Input: part model. Units: mm. Frame: model coordinates. A direction names the side the tool comes from. Round coordinates to 2 decimals unless told otherwise and drop trailing zeros. Write each loop counter-clockwise with the first axis right and the second up, starting at its lowest first coordinate (ties: lowest second). Pieces come first, ordered by that corner, then holes. Notation, with made-up numbers: (58, 24.25) - (116, 24.25) arc R14 ccw to (116, 28.25) - close; hole circle Ø5 at (-9, 30.5). An arc over 180 degrees is marked (long way). One line per item, written item: value. Start each with the question number.
```python
from build123d import *

# Parameters (mm, degrees)
BOSS_EXTRUDE1_DEPTH     = 6.35
F_3_8_CLEARANCE_HOLE1_D = 10.0838
BODY_MOVE_COPY2_ANGLE   = 90
F_1_4_CLEARANCE_HOLE1_D = 6.7564
SKETCH6_W               = 11.2395
SKETCH6_H               = 11.2395
CUT_EXTRUDE1_DEPTH      = 6.8326
F_3_8_CLEARANCE_HOLE3_D = 10.0838
FILLET1_R               = 3.175
F_3_8_CLEARANCE_HOLE2_D = 13.97


with BuildPart() as part:
    # Sketch2 → Boss-Extrude1 (new, symmetric)
    with BuildSketch(Plane.XY):
        Polygon((-25.4, -25.4), (25.4, -25.4), (25.4, 50.8), (12.7, 76.2), (-12.7, 76.2), (-25.4, 50.8), align=None)
    extrude(amount=BOSS_EXTRUDE1_DEPTH, both=True)

    # 3/8 Clearance Hole1 (through all)
    with Locations(Plane.XY.offset(6.35)):
        with Locations((0, 0), (0, 57.15)):
            Hole(F_3_8_CLEARANCE_HOLE1_D / 2)


with BuildPart() as body_2:
    # uxcell-FR6ZZ: read off the stored shape, not the designer's step
    # uxcell-FR6ZZ outline → uxcell-FR6ZZ (revolve)
    with BuildSketch(Plane(origin=(-48.38860798, 0, 0), x_dir=(1, 0, 0), z_dir=(0, 0, 1))):
        Polygon((12.430125, 12.468326067), (4.7625, 12.468326067), (4.7625, 4.054576067), (11.2395, 4.054576067), (11.2395, 9.213951067), (11.636375, 9.610826067), (12.430125, 9.610826067), align=None)
    revolve(axis=Axis((-48.38860798, 0, 0), (0, 1, 0)))


with BuildPart() as body_2_1:
    # Body-Move/Copy2: read off the stored shape, not the designer's step
    # Body-Move/Copy2: moved
    add(body_2.part.moved(Location((48.388608, -6.1183261, 0))).rotate(Axis((0, 0, 0), (1, 0, 0)), BODY_MOVE_COPY2_ANGLE))


with BuildPart() as part_1:
    add(part.part)

    # Combine1: cut body 2
    add(body_2_1.part, mode=Mode.SUBTRACT)

    # 1/4 Clearance Hole1 (through all)
    with Locations(Plane.XY.offset(6.35)):
        with Locations((-15.875, 15.875), (15.875, 15.875), (15.875, -15.875), (-15.875, -15.875)):
            Hole(F_1_4_CLEARANCE_HOLE1_D / 2)

    # Sketch6 → Cut-Extrude1 (cut)
    with BuildSketch(Plane.XY.offset(6.35)):
        with Locations((-15.875, 15.875)):
            Rectangle(SKETCH6_W, SKETCH6_H)
    cut_extrude1 = extrude(amount=-CUT_EXTRUDE1_DEPTH, mode=Mode.SUBTRACT)

    # Sketch-Pattern1: Cut-Extrude1 at 3 more places
    with Locations((0, -31.75, 0), (31.75, -31.75, 0), (31.75, 0, 0)):
        add(cut_extrude1, mode=Mode.SUBTRACT)

    # 3/8 Clearance Hole3 (through all)
    with Locations(Plane(origin=(0, 0, -6.35), x_dir=(-1, 0, 0), z_dir=(0, 0, -1))):
        with Locations((0, 57.15)):
            Hole(F_3_8_CLEARANCE_HOLE3_D / 2)

    # Fillet1
    fillet1_edges = [part_1.edges().sort_by_distance(p)[0] for p in [
        (-25.4, 50.8, 0),
        (-12.7, 76.2, 0),
        (12.7, 76.2, 0),
        (25.4, 50.8, 0),
        (25.4, -25.4, 0),
        (-25.4, -25.4, 0),
    ]]
    fillet(fillet1_edges, radius=FILLET1_R)

    # 3/8 Clearance Hole2 (through all)
    with Locations(Plane.XY.offset(6.35)):
        with Locations((0, 0)):
            Hole(F_3_8_CLEARANCE_HOLE2_D / 2)


solid = part_1.part
```
Q1. Cut plane B-B, the plane y = 57.15. Output: boundary loops of the cut face in (x, z) (3 decimals), and give its area (3 significant figures).
Q2. Contact query for flat-ended pins moving along their axis: pin 1 Ø9 at (x, y) = (15.875, 15.875) entering from -Z; pin 2 Ø4 at (x, y) = (-15.875, -15.875) entering from +Z; pin 3 Ø11 at (x, y) = (5.5, -2) entering from +Z; pin 4 Ø1.5 at (y, z) = (64, -1.5) entering from -X (3 decimals). Output: stop coordinate, or through.
Q3. Cut plane C-C, the plane y = -18. Output: boundary loops of the cut face in (x, z), and give its area (3 significant figures).
Q4. Material intervals for probe 1 along Y at (x, z) = (0, 3.75); probe 2 along Y at (x, z) = (0, -3.35) (3 decimals); probe 3 along Z at (x, y) = (-10.5, -6), sorted ascending. Write a range as from..to.
Q5. Cut plane A-A, the plane x = 0. Count the separate pieces of the cut face and the enclosed holes in it, and give its area (3 significant figures).
Q6. Access query for faces 1 (the flat face through (19.4, 62.8, 0.1)), 2 (the flat face through (10.255, -16, 3)). Directions: +Z, -Z, +X, -X, +Y, -Y. A direction counts if a zero-diameter tool reaches every point of the face in a straight line with its end or side. Return the directions, or none.
Q7. Cut plane D-D, the plane z = -4.75. Output: boundary loops of the cut face in (x, y) (3 decimals), and give its area (3 significant figures).
Q8. Pull-direction query (X, two-part tool) for faces 3 (the flat face through (0, -25.4, 0)), 4 (the flat face through (0.2, -7.3, -2.064)), 5 (the flat face through (-25.4, 14, 0)); classes: pulls with the +X half, pulls with the -X half, needs draft (parallel to the pull), parting line crosses it, or undercut.
A:
1. outline: (-22.225, -6.35) - (-5.042, -6.35) - (-5.042, 6.35) - (-22.225, 6.35) - close; (5.042, -6.35) - (22.225, -6.35) - (22.225, 6.35) - (5.042, 6.35) - close
1. area: 436 mm²
2. pin 1: stops at z = -6.35
2. pin 2: passes through
2. pin 3: stops at z = 3.21
2. pin 4: stops at x = -19.175
3. outline: (-25.4, -6.35) - (-18.5, -6.35) - (-18.5, -0.48) - (-21.49, -0.48) - (-21.49, 6.35) - (-25.4, 6.35) - close; (-13.25, -6.35) - (13.25, -6.35) - (13.25, -0.48) - (10.26, -0.48) - (10.26, 6.35) - (-10.26, 6.35) - (-10.26, -0.48) - (-13.25, -0.48) - close; (18.5, -6.35) - (25.4, -6.35) - (25.4, 6.35) - (21.49, 6.35) - (21.49, -0.48) - (18.5, -0.48) - close
3. area: 430 mm²
4. probe 1: y = -25.4..-12.43, 12.43..52.11, 62.19..76.2
4. probe 2: y = -25.4..-6.985, 6.985..52.108, 62.192..76.2
4. probe 3: z = -6.35..3.49
5. separate pieces: 3
5. enclosed holes: 0
5. area: 906 mm²
6. face 1: +Z, -Z, +X, +Y
6. face 2: +Z
7. outline: (-25.4, -22.225) arc R3.175 ccw to (-22.225, -25.4) - (22.225, -25.4) arc R3.175 ccw to (25.4, -22.225) - (25.4, 50.05) arc R3.175 ccw to (25.065, 51.47) - (13.578, 74.445) arc R3.175 ccw to (10.738, 76.2) - (-10.738, 76.2) arc R3.175 ccw to (-13.578, 74.445) - (-25.065, 51.47) arc R3.175 ccw to (-25.4, 50.05) - close; hole circle Ø6.756 at (-15.875, -15.875); hole circle Ø6.756 at (-15.875, 15.875); hole circle Ø13.97 at (0, 0); hole circle Ø10.084 at (0, 57.15); hole circle Ø6.756 at (15.875, -15.875); hole circle Ø6.756 at (15.875, 15.875)
7. area: 4,460 mm²
8. face 3: needs draft
8. face 4: undercut
8. face 5: pulls with the -X half
